from build123d import *

# Parameters (mm, degrees)
ESBO_O2_R                  = 100
ESBO_O2_R_2                = 95
RESSALTO_EXTRUS_O2_DEPTH   = 1400
CORTE_EXTRUS_O1_DEPTH      = 1408.124727947
CORTE_EXTRUS_O1_DEPTH_BACK = 1408.124727947
ESBO_O3_R                  = 25
ESBO_O4_W                  = 14.042229064
ESBO_O4_H                  = 57.796016078
CORTE_EXTRUS_O2_DEPTH      = 92.5
ESBO_O5_R                  = 20
CORTE_EXTRUS_O3_DEPTH      = 185


with BuildPart() as part:
    # Esboço2 → Ressalto-extrusão2 (new body)
    with BuildSketch(Plane.XY):
        Circle(ESBO_O2_R)
        Circle(ESBO_O2_R_2, mode=Mode.SUBTRACT)
    extrude(amount=RESSALTO_EXTRUS_O2_DEPTH)

    # Esboço3 → Corte-extrusão1 (cut, two sides: drawn at the far end of the back side and taken through both)
    with BuildSketch(Plane(origin=(0, 0, 0), x_dir=(0, 0, -1), z_dir=(1, 0, 0)).offset(-CORTE_EXTRUS_O1_DEPTH_BACK)):
        with Locations((-700, 0)):
            Circle(ESBO_O3_R)
    extrude(amount=CORTE_EXTRUS_O1_DEPTH + CORTE_EXTRUS_O1_DEPTH_BACK, mode=Mode.SUBTRACT)

    # Esboço4 → Corte-extrusão2 (cut, symmetric)
    with BuildSketch(Plane(origin=(0, 0, 0), x_dir=(0, 0, -1), z_dir=(1, 0, 0))):
        with Locations((-700, 0)):
            Rectangle(ESBO_O4_W, ESBO_O4_H)
    extrude(amount=CORTE_EXTRUS_O2_DEPTH, both=True, mode=Mode.SUBTRACT)

    # Esboço5 → Corte-extrusão3 (cut)
    with BuildSketch(Plane(origin=(0, 0, 0), x_dir=(0, 0, -1), z_dir=(1, 0, 0))):
        with Locations(Location((-137.826137531, 0, 0), (0, 0, 180))):
            Circle(ESBO_O5_R)
    extrude(amount=CORTE_EXTRUS_O3_DEPTH, mode=Mode.SUBTRACT)


solid = part.part
Read the model definition and answer for the solid it produces. Units are mm, in the model's axes. A direction names the side the tool comes from. Round coordinates to 2 decimals unless told otherwise and drop trailing zeros. Write each loop counter-clockwise with the first axis right and the second up, starting at its lowest first coordinate (ties: lowest second). Pieces come first, ordered by that corner, then holes. Notation, with made-up numbers: (68.25, 16.5) - (116.25, 16.5) arc R31 ccw to (116.25, 40.5) - close; hole circle Ø2 at (0, 10.25). An arc over 180 degrees is marked (long way). Use a Markdown table: item, result.
(1) Straight lines are drawn through the part: line 1 along X through (y, z) = (0, 926); line 2 along Y through (x, z) = (37.5, 72). For each, find the intervals that lie inside material, in ascending order. Write a range as [from, to].
Reported:
| item | result |
|---|---|
| line 1 | [-100, -95], [95, 100] |
| line 2 | [-92.7, -87.29], [87.29, 92.7] |
(2) Each of these flat-tipped pins is pushed along its axis until it touches: pin 1 Ø6 at (x, z) = (35.5, 1126) entering from +Y; pin 2 Ø5 at (y, z) = (-50, 1054.5) entering from +X; pin 3 Ø5.5 at (y, z) = (26.5, 701) entering from +X. Where does it stop, or does it pass through?
Reported:
| item | result |
|---|---|
| pin 1 | y = 94.57 |
| pin 2 | x = 88 |
| pin 3 | x = 96.88 |
(3) The part is cut by section B-B (y = -47). Write down the section's boundary in (x, z).
Reported:
| item | result |
|---|---|
| outline | (-88.27, 0) - (-82.56, 0) - (-82.56, 1400) - (-88.27, 1400) - close; (82.56, 0) - (88.27, 0) - (88.27, 1400) - (82.56, 1400) - close |
(4) The mould has two halves that part along Y. Classify faces 3 (the cylindrical face through (95.38, 30.04, 690.2)), 4 (the cylindrical face through (-96.017, -24.406, 705.42)), 5 (the flat face through (88, -37, 0)): released by +Y, released by -Y, zero draft, split by the parting line, or undercut.
Reported:
| item | result |
|---|---|
| face 3 | split by the parting line |
| face 4 | undercut |
| face 5 | zero draft |
(5) Which of the six approach directions +Z, -Z, +X, -X, +Y, -Y give full straight-line access (tool end or side, diameter ignored) to faces 1 (the flat face through (88, -37, 1400)), 2 (the cylindrical face through (96.39, 7.66, 156.3))?
Reported:
| item | result |
|---|---|
| face 1 | +Z, +X, -X, +Y, -Y |
| face 2 | +X |
(6) The part is cut by section A-A (x = 0). Write down the section's boundary in (y, z).
Reported:
| item | result |
|---|---|
| outline | (-100, 0) - (-95, 0) - (-95, 1400) - (-100, 1400) - close; (95, 0) - (100, 0) - (100, 1400) - (95, 1400) - close |
(7) The part is cut by section C-C (z = 277). Write down the section's boundary in (x, y), then the cut area to 3 significant figures.
Reported:
| item | result |
|---|---|
| outline | circle Ø200 at (0, 0); hole circle Ø190 at (0, 0) |
| area | 3,060 mm2 |
